Work out the finished part from the listing and answer in its coordinate system (mm). Face numbers are marked on the shaded views. A direction names the side the tool comes from. Coordinates: 2 decimals unless noted, no trailing zeros. Order: outer loops, then holes, each group sorted by start corner. A loop starts at its lowest first (then second) coordinate and runs counter-clockwise, first axis right, second up. Notation, with made-up numbers: M 67.25,32.25 L 112.25,32.25 A27 cw 112.25,55.25 Z; hole C 8.25,61.5 d6. An arc over 180 degrees is marked long. Use a Markdown table: item, result.
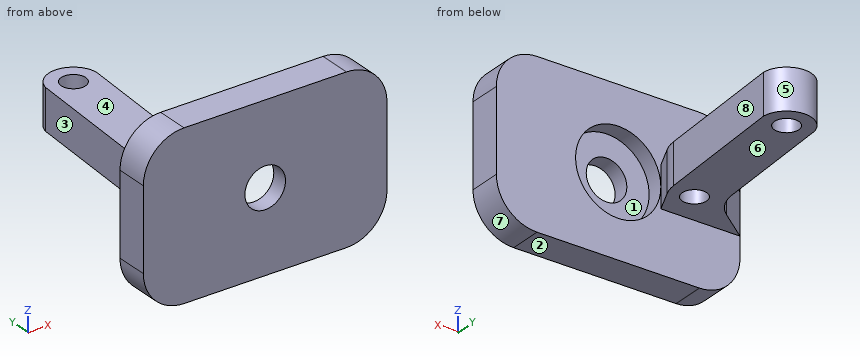
from build123d import *

# Parameters (mm, degrees)
SKETCH1_W           = 30
SKETCH1_H           = 20
BOSS_EXTRUDE1_DEPTH = 4
SKETCH2_R           = 5.25
CUT_EXTRUDE1_DEPTH  = 2
SKETCH3_R           = 2.5
CUT_EXTRUDE2_DEPTH  = 5
SKETCH4_R           = 1.5
BOSS_EXTRUDE2_DEPTH = 2.5
FILLET1_R           = 5
FILLET2_R           = 5


with BuildPart() as part:
    # Sketch1 → Boss-Extrude1 (new body)
    with BuildSketch(Plane(origin=(0, 0, 0), x_dir=(1, 0, 0), z_dir=(0, 1, 0))):
        Rectangle(SKETCH1_W, SKETCH1_H)
    extrude(amount=BOSS_EXTRUDE1_DEPTH)

    # Sketch2 → Cut-Extrude1 (cut)
    with BuildSketch(Plane(origin=(0, 4, 0), x_dir=(1, 0, 0), z_dir=(0, 1, 0))):
        Circle(SKETCH2_R)
    extrude(amount=-CUT_EXTRUDE1_DEPTH, mode=Mode.SUBTRACT)

    # Sketch3 → Cut-Extrude2 (cut, through all)
    with BuildSketch(Plane(origin=(0, 4, 0), x_dir=(1, 0, 0), z_dir=(0, 1, 0))):
        Circle(SKETCH3_R)
    extrude(amount=-CUT_EXTRUDE2_DEPTH, mode=Mode.SUBTRACT)

    # Sketch4 → Boss-Extrude2 (add, symmetric)
    with BuildSketch(Plane.XY):
        with BuildLine():
            Line((-15, 4), (-9.492692151, 8.218800623))
            Line((-9.492692151, 8.218800623), (-8.237245547, 26.172523512))
            ThreePointArc((-8.237245547, 26.172523512), (-5.067133546, 28.50047615), (-2.251861245, 25.75398467))
            Line((-2.251861245, 25.75398467), (-3.507307849, 7.800261781))
            Line((-3.507307849, 7.800261781), (-5.25, 4))
            Line((-5.25, 4), (-15, 4))
        make_face()
        with Locations((-6.5, 8.009531202)):
            Circle(SKETCH4_R, mode=Mode.SUBTRACT)
        with Locations((-5.279261709, 25.466902082)):
            Circle(SKETCH4_R, mode=Mode.SUBTRACT)
    extrude(amount=BOSS_EXTRUDE2_DEPTH, both=True)

    # Fillet1
    fillet1_edges = [part.edges().sort_by_distance(p)[0] for p in [
        (-9.492692151, 8.218800623, 0),
        (-3.507307849, 7.800261781, 0),
    ]]
    fillet(fillet1_edges, radius=FILLET1_R)

    # Fillet2
    fillet2_edges = [part.edges().sort_by_distance(p)[0] for p in [
        (15, 2, 10),
        (-15, 2, 10),
        (-15, 2, -10),
        (15, 2, -10),
    ]]
    fillet(fillet2_edges, radius=FILLET2_R)


solid = part.part
1. Section D-D on x = 4.25 is taken. Determine the outline of the cut face in (y, z).
Answers below:
| item | result |
|---|---|
| outline | M 0,-10 L 4,-10 L 4,-3.08 L 2,-3.08 L 2,3.08 L 4,3.08 L 4,10 L 0,10 Z |
2. Flat-ended cylindrical pins translate along their axes: P1, Ø10, axis at y = 23.5, z = 0.5, coming from the +X side; P2, Ø10, axis at x = -7.5, y = 18.5, coming from the +Z side; P3, Ø10, axis at x = 7, z = 4, coming from the +Y side. Find the tip coordinate at first contact, or state that the pin passes through.
Answers below:
| item | result |
|---|---|
| P1 | x = -2.25 |
| P2 | z = 2.5 |
| P3 | y = 4 |
3. For the marked faces 4, 5, 6, 7 and 8, determine the directions among +Z, -Z, +X, -X, +Y, -Y from which every point of the face is accessible in a straight line to the end or side of a thin tool.
Answers below:
| item | result |
|---|---|
| face 4 | +Z, +X, -X, +Y |
| face 5 | +Z, -Z, +Y |
| face 6 | -Z, +X, -X, +Y |
| face 7 | -Z, +X, +Y, -Y |
| face 8 | +Z, -Z, +X |
4. Section B-B on z = -0.75 is taken. Determine the outline of the cut face in (x, y), then the cut area to 3 significant figures.
Answers below:
| item | result |
|---|---|
| outline | M -15,0 L -2.38,0 L -2.38,2 L -5.2,2 L -5.2,4 L -5.25,4 L -3.89,6.97 A5 ccw -3.44,8.71 L -2.25,25.75 A3.04 ccw -8.24,26.17 L -9.34,10.47 A5 cw -11.28,6.85 L -15,4 Z; M 2.38,0 L 15,0 L 15,4 L 5.2,4 L 5.2,2 L 2.38,2 Z; hole C -6.5,8.01 d3; hole C -5.28,25.47 d3 |
| area | 228 mm² |
5. Section C-C on z = -4.5 is taken. Determine the outline of the cut face in (x, y).
Answers below:
| item | result |
|---|---|
| outline | M -15,0 L 15,0 L 15,4 L 2.7,4 L 2.7,2 L -2.7,2 L -2.7,4 L -15,4 Z |
6. For a pull along Z with two mould halves and no side action, classify the marked faces 1, 2 and 3 as +Z half, -Z half, draft (parallel to the pull), parting line (faces both ways), or undercut.
Answers below:
| item | result |
|---|---|
| face 1 | undercut |
| face 2 | -Z half |
| face 3 | draft |
7. Find the intervals of material crossed by probe 1 along Z at (x, y) = (0, 3.45); probe 2 along X at (y, z) = (2.9, 0); probe 3 along Y at (x, z) = (-2.25, 5.75), in increasing order.
Answers below:
| item | result |
|---|---|
| probe 1 | -10 to -5.25, 5.25 to 10 |
| probe 2 | -15 to -5.25, 5.25 to 15 |
| probe 3 | 0 to 4 |
8. Section A-A on x = 0 is taken. Determine the outline of the cut face in (y, z).
Answers below:
| item | result |
|---|---|
| outline | M 0,-10 L 4,-10 L 4,-5.25 L 2,-5.25 L 2,-2.5 L 0,-2.5 Z; M 0,2.5 L 2,2.5 L 2,5.25 L 4,5.25 L 4,10 L 0,10 Z |
